Geometry check sheet. Reference: the model listing, model coordinates, mm. A direction names the side the tool comes from. Coordinates: 2 decimals unless noted, no trailing zeros. Order: outer loops, then holes, each group sorted by start corner. A loop starts at its lowest first (then second) coordinate and runs counter-clockwise, first axis right, second up. Notation, with made-up numbers: (44.5, 57.5) - (103.5, 57.5) arc R26 ccw to (103.5, 95.5) - close; hole circle Ø2 at (18, -14). An arc over 180 degrees is marked (long way). One line per item, written item: value. Start each with the question number.
```python
from build123d import *

# Parameters (mm, degrees)
F0_R     = 5.534072
F0_R_2   = 5.262589
F1_DEPTH = 12.7
F2_R     = 4.5907
F2_R_2   = 4.594767
F3_DEPTH = 25.4


with BuildPart() as f1:
    # F0 (on Front) → F1 (new body)
    with BuildSketch(Plane.XZ):
        with BuildLine():
            ThreePointArc((16.002001, 24.957247), (-8.808441, 49.767689), (-33.618882, 24.957247))
            Line((-33.618882, 24.957247), (-33.618882, -36.408219))
            ThreePointArc((-33.618882, -36.408219), (-8.808441, -61.218661), (16.002001, -36.408219))
            Line((16.002001, -36.408219), (16.002001, 24.957247))
        make_face()
        with Locations((-8.808441, -47.565579)):
            Circle(F0_R, mode=Mode.SUBTRACT)
        with Locations((-8.808441, 37.582681)):
            Circle(F0_R_2, mode=Mode.SUBTRACT)
    extrude(amount=F1_DEPTH)

    # F2 (on Front) → F3 (join)
    with BuildSketch(Plane.XZ):
        with BuildLine():
            ThreePointArc((4.551028, 17.910495), (-7.193559, 25.868808), (-18.938147, 17.910495))
            Line((-18.938147, 17.910495), (-18.938147, -28.480623))
            ThreePointArc((-18.938147, -28.480623), (-7.193559, -36.411624), (4.551028, -28.480623))
            Line((4.551028, -28.480623), (4.551028, 17.910495))
        make_face()
        with Locations((-7.193559, -23.750164)):
            Circle(F2_R, mode=Mode.SUBTRACT)
        with Locations((-7.193559, 13.223535)):
            Circle(F2_R_2, mode=Mode.SUBTRACT)
    extrude(amount=F3_DEPTH)


solid = f1.part
```
Q1. Cross-section at C-C, the plane y = -19.5. Enter the section's corners in (x, z), and give its area (3 significant figures).
Q2. Material ranges on probe 1 along Z at (x, y) = (-11, -21.25); probe 2 along X at (y, z) = (-16.5, -5.5); probe 3 along Y at (x, z) = (-2.5, 31.5), recorded low to high.
Q3. Release check for a two-part mould opening along Z. For faces 4 (the flat face through (4.551, -19, -6)), 5 (the cylindrical face through (-9.354, -6.261, -61.213)), 6 (the cylindrical face through (-8.19, -18.96, 8.74)) record: released by +Z, released by -Z, zero draft, split by the parting line, or undercut.
Q4. Gauge pin test, flat ends, axial feed: P1, Ø4, axis at x = -5, y = -12, coming from the -Z side; P2, Ø10, axis at x = 5.5, y = -10, coming from the -Z side; P3, Ø12, axis at x = -5.5, y = -18.5, coming from the +Z side. Record the tip position at first contact, or that the pin passes through.
Q5. Cross-section at D-D, the plane x = -25. Enter the section's corners in (y, z).
Q6. Set-up check for faces 1 (the cylindrical face through (-7.4, -18.96, -36.41)), 2 (the cylindrical face through (-6.983, -18.961, 25.867)), 3 (the flat face through (-7, -12.7, -24)): record each of +Z, -Z, +X, -X, +Y, -Y from which the full face is reachable in a straight line by a thin tool's end or side.
Q7. Cross-section at B-B, the plane z = -10. Enter the section's corners in (x, y), and give its area (4 significant figures).
Q8. Cross-section at A-A, the plane z = 41. Enter the section's corners in (x, y), and give its area (3 significant figures).
Check result:
1. outline: (-18.94, -28.48) arc R12.66 ccw to (4.55, -28.48) - (4.55, 17.91) arc R12.65 ccw to (-18.94, 17.91) - close; hole circle Ø9.19 at (-7.19, 13.22); hole circle Ø9.18 at (-7.19, -23.75)
1. area: 1,230 mm2
2. probe 1: z = -35.83 to -26.32, -21.18 to 10.65, 15.8 to 25.28
2. probe 2: x = -18.94 to 4.55
2. probe 3: y = -12.7 to 0
3. face 4: zero draft
3. face 5: released by -Z
3. face 6: undercut
4. P1: stops at z = -61.15
4. P2: stops at z = -59.41
4. P3: stops at z = 49.7
5. outline: (-12.7, -55.21) - (0, -55.21) - (0, 43.76) - (-12.7, 43.76) - close
6. face 1: -Z, -Y
6. face 2: +Z, -Y
6. face 3: -Y
7. outline: (-33.62, -12.7) - (-18.94, -12.7) - (-18.94, -25.4) - (4.55, -25.4) - (4.55, -12.7) - (16, -12.7) - (16, 0) - (-33.62, 0) - close
7. area: 928.5 mm2
8. outline: (-27.73, -12.7) - (-12.81, -12.7) - (-12.81, 0) - (-27.73, 0) - close; (-4.81, -12.7) - (10.12, -12.7) - (10.12, 0) - (-4.81, 0) - close
8. area: 379 mm2
